Geometry check sheet. Reference: the model listing, model coordinates, mm. A direction names the side the tool comes from. Coordinates: 2 decimals unless noted, no trailing zeros. Write each loop counter-clockwise with the first axis right and the second up, starting at its lowest first coordinate (ties: lowest second). Pieces come first, ordered by that corner, then holes. Notation, with made-up numbers: (-27, -23.5) -> (-13, -23.5) arc R24 ccw to (-13, 6.5) -> close; hole circle Ø5 at (-34.5, 89). An arc over 180 degrees is marked (long way). Answer in a Markdown table with one row per item. Add a question column.
Q1. Gauge pin test, flat ends, axial feed: P1, Ø4, axis at x = 0.5, z = 4, coming from the -Y side; P2, Ø4, axis at x = 0.5, z = 5, coming from the +Y side. Record the tip position at first contact, or that the pin passes through.
Q2. Section check A-A, the plane x = 0. Record the boundary of the cut face in (y, z) (3 decimals).
Q3. Tool access check on faces 1 (the face through (-0.434, 2.387, 3.429)), 2 (the face through (6.5, 3, 5)), 3 (the face through (0, 5, 7.95)). Record the directions out of +Z, -Z, +X, -X, +Y, -Y that give a thin tool (end or side, any length) a straight path to the whole face; none if there is none.
Q4. Release check for a two-part mould opening along Z. For faces 4 (the face through (-0.099, 2.282, 5.394)), 5 (the face through (0, 3, 8.75)), 6 (the face through (-6.5, 3, 5)), 7 (the face through (0, 3, 1.95)) record: pulls with the +Z half, pulls with the -Z half, needs draft (parallel to the pull), parting line crosses it, or undercut.
Q5. Section check B-B, the plane y = 2.25. Record the boundary of the cut face in (x, z) (3 decimals).
Q6. Thickness scan on line 1 (Z direction, x = 0, y = 3.65) (3 decimals); line 2 (X direction, y = 2.25, z = 3.9) (3 decimals); line 3 (Y direction, x = 0, z = 3) (3 decimals). Record the ranges inside material, lowest first.
Q7. Section check C-C, the plane z = 5.25. Record the boundary of the cut face in (x, y).
Autodesk Inventor part; units mm, degrees
ref_plane "YZ Plane" through (0, 0, 0) normal (1, 0, 0) x (0, 1, 0)
ref_plane "XZ Plane" through (0, 0, 0) normal (0, 1, 0) x (-1, 0, 0)
ref_plane "XY Plane" through (0, 0, 0) normal (0, 0, 1) x (1, 0, 0)
sketch "Skizze1" plane through (0, 0, 0) normal (0, 1, 0) x (-1, 0, 0)
  line L0 (-6.5, -8.75) -> (6.5, -8.75)
  line L1 (6.5, -8.75) -> (6.5, 8.75)
  line L2 (6.5, 8.75) -> (-6.5, 8.75)
  line L3 (-6.5, 8.75) -> (-6.5, -8.75)
  line L4 (-6.5, -8.75) -> (6.5, 8.75) construction
  line L5 (6.5, -8.75) -> (-6.5, 8.75) construction
  point P0 (0, 0)
  dimension "d0" = 13
  dimension "d1" = 17.5
extrude "Extrusion1" add sketch "Skizze1" along normal blind 5.5
sketch "Skizze2" plane through (0, 5.5, 0) normal (0, 1, 0) x (1, 0, 0)
  line L0 (-6.5, 8.75) -> (-6.5, -8.75)
  line L1 (-6.5, -8.75) -> (6.5, -8.75)
  line L2 (6.5, -8.75) -> (6.5, 8.75)
  line L3 (6.5, 8.75) -> (-6.5, 8.75)
  line L4 (3.75, -1.95) -> (-3.75, -1.95)
  line L5 (-3.75, -1.95) -> (-3.75, -7.95)
  line L6 (-3.75, -7.95) -> (3.75, -7.95)
  line L7 (3.75, -7.95) -> (3.75, -1.95)
  line L8 (3.75, -1.95) -> (-3.75, -7.95) construction
  line L9 (-3.75, -1.95) -> (3.75, -7.95) construction
  point P0 (0, 0)
  point P1 (0, -4.95)
  dimension "d4" = 7.5
  dimension "d5" = 6
  dimension "d17" = 0.8
extrude "Extrusion2" cut sketch "Skizze2" against normal blind 1 contours L7 L6 L5 L4
sketch "Skizze3" plane through (0, 5.5, 0) normal (0, 1, 0) x (1, 0, 0)
  line L0 (-6.5, 8.75) -> (-6.5, -8.75)
  line L1 (3.75, -7.95) -> (-3.75, -7.95)
  line L2 (-3.75, -7.95) -> (-3.75, -1.95)
  line L3 (-3.75, -1.95) -> (3.75, -1.95)
  line L4 (3.75, -1.95) -> (3.75, -7.95)
  line L5 (-6.5, 8.75) -> (-6.5, -8.75)
  line L6 (-6.5, -8.75) -> (6.5, -8.75)
  line L7 (6.5, -8.75) -> (6.5, 8.75)
  line L8 (6.5, 8.75) -> (-6.5, 8.75)
  line L9 (6.5, -8.75) -> (6.5, 8.75)
  line L10 (-6.5, -8.75) -> (6.5, -8.75)
  line L11 (6.5, -8.75) -> (6.5, -1.95)
  line L12 (6.5, -1.95) -> (-6.5, -1.95)
  line L13 (-6.5, -1.95) -> (-6.5, -8.75)
  point P0 (0, 0)
  point P1 (-6.5, -1.95)
  dimension "d8" = 6.8
extrude "Extrusion3" cut sketch "Skizze3" against normal blind 0.1 contours L12 L2 L1 L4 L7 L6 L0
sketch "Skizze4" plane through (6.5, 0, -8.75) normal (0, 0, -1) x (-1, 0, 0)
  line L0 (0, 0) -> (13, 0)
  line L1 (13, 0) -> (13, 5.5)
  line L2 (0, 5.5) -> (13, 5.5)
  line L3 (0, 0) -> (0, 5.5)
  line L4 (10.15, 4.75) -> (2.85, 4.75)
  line L5 (2.85, 4.75) -> (2.85, 0.75)
  line L6 (2.85, 0.75) -> (10.15, 0.75)
  line L7 (10.15, 0.75) -> (10.15, 4.75)
  line L8 (10.15, 4.75) -> (2.85, 0.75) construction
  line L9 (2.85, 4.75) -> (10.15, 0.75) construction
  point P0 (6.5, 0)
  point P1 (6.5, 2.75)
  dimension "d11" = 7.3
  dimension "d12" = 4
extrude "Extrusion4" cut sketch "Skizze4" against normal blind 0.1 contours L7 L6 L5 L4
sketch "Skizze5" plane through (0, 5.5, 0) normal (0, 1, 0) x (1, 0, 0)
  line L0 (-6.5, -1.95) -> (6.5, -1.95)
  line L1 (6.5, -1.95) -> (6.5, 8.75)
  line L2 (6.5, 8.75) -> (-6.5, 8.75)
  line L3 (-6.5, 8.75) -> (-6.5, -1.95)
  point P0 (0, 0)
extrude "Extrusion5" cut sketch "Skizze5" against normal blind 10
sketch "Skizze6" plane through (0, 4.5, 0) normal (0, 1, 0) x (1, 0, 0)
  line L0 (-3.75, -7.95) -> (-3.75, -1.95)
  line L1 (3.75, -7.95) -> (-3.75, -7.95)
  line L2 (3.75, -1.95) -> (3.75, -7.95)
  line L3 (-3.75, -1.95) -> (3.75, -1.95)
  circle A0 centre (0, -4.95) radius 0.455
  point P0 (0, 0)
extrude "Extrusion6" cut sketch "Skizze6" against normal blind 10 contours A0
sketch "Skizze7" plane through (6.5, 0, 1.95) normal (0, 0, -1) x (-1, 0, 0)
  line L0 (13, 5.4) -> (10.25, 5.4)
  line L1 (10.25, 5.4) -> (10.25, 4.5)
  line L2 (10.25, 4.5) -> (2.75, 4.5)
  line L3 (2.75, 5.4) -> (2.75, 4.5)
  line L4 (2.75, 5.4) -> (0, 5.4)
  line L5 (0, 0) -> (0, 5.4)
  line L6 (13, 0) -> (0, 0)
  line L7 (13, 5.4) -> (13, 0)
  line L8 (6.045, 4.5) -> (6.955, 4.5)
  line L9 (2.75, 4.5) -> (10.25, 4.5)
  line L10 (10.25, 4.5) -> (2.75, 4.5)
  line L11 (6.955, 4.5) -> (6.955, 0)
  line L12 (6.045, 4.5) -> (6.045, 0)
  circle A0 centre (6.5, 2.25) radius 0.455
  point P0 (6.5, 0)
extrude "Extrusion7" cut sketch "Skizze7" against normal up to surface contours A0
properties part number "00_HuaweiP30_Telelens_prismonly"
Calculated:
| question | item | result |
|---|---|---|
| 1 | P1 | stops at y = 0 |
| 1 | P2 | stops at y = 4.5 |
| 2 | outline | (0, 1.95) -> (1.795, 1.95) -> (1.795, 4.495) -> (0, 4.495) -> close; (0, 5.405) -> (4.5, 5.405) -> (4.5, 7.95) -> (5.4, 7.95) -> (5.4, 8.75) -> (0, 8.75) -> close; (2.705, 1.95) -> (4.5, 1.95) -> (4.5, 4.495) -> (2.705, 4.495) -> close |
| 3 | face 1 | -Z |
| 3 | face 2 | +Z, -Z, +X, +Y, -Y |
| 3 | face 3 | -Z, +Y |
| 4 | face 4 | undercut |
| 4 | face 5 | pulls with the +Z half |
| 4 | face 6 | needs draft |
| 4 | face 7 | pulls with the -Z half |
| 5 | outline | (-6.5, 1.95) -> (-0.455, 1.95) -> (-0.455, 4.95) arc R0.455 cw to (0.455, 4.95) -> (0.455, 1.95) -> (6.5, 1.95) -> (6.5, 8.75) -> (-6.5, 8.75) -> close |
| 6 | line 1 | z = 1.95 to 4.495, 5.405 to 8.75 |
| 6 | line 2 | x = -6.5 to -0.455, 0.455 to 6.5 |
| 6 | line 3 | y = 0 to 1.795, 2.705 to 4.5 |
| 7 | outline | (-6.5, 0) -> (-0.34, 0) -> (-0.34, 4.5) -> (-3.75, 4.5) -> (-3.75, 5.4) -> (-6.5, 5.4) -> close; (0.34, 0) -> (6.5, 0) -> (6.5, 5.4) -> (3.75, 5.4) -> (3.75, 4.5) -> (0.34, 4.5) -> close |
